Work out the finished part from the listing and answer in its coordinate system (mm). Face numbers are marked on the shaded views. A direction names the side the tool comes from. Give positions to 0.01 mm unless a question says otherwise; leave off trailing zeros. Loops run counter-clockwise (first coordinate to the right, second up) from the corner with the lowest first, then second, coordinate; pieces in that order, holes last. Notation, with made-up numbers: (54.5, 68.5) - (66.5, 68.5) arc R8 cw to (66.5, 80.5) - close; hole circle Ø4 at (60, 33). An arc over 180 degrees is marked (long way). One line per item, written item: value.
from build123d import *

# Parameters (mm, degrees)
F3_R          = 2.5
F4_DEPTH      = 42.28
F4_DEPTH_BACK = 29.68
F5_DEPTH      = 30
F5_DEPTH_BACK = 29.68
F3_W          = 18.04
F3_H          = 15.5
F3_R_2        = 5.32
F8_DEPTH      = 30
F9_START      = -20
F1_R          = 5.32
F1_R_2        = 3.41
F9_DEPTH      = 10
F10_R         = 4
F12_DEPTH     = 56.231
F14_DEPTH     = 74.271


# Not quite as in the source:
# - a feature of the source that left no trace in its solid (it failed there, or was rolled back) is left out


with BuildPart() as f4:
    # F3 (on Front) → F4 (new body, two sides)
    with BuildSketch(Plane.XZ) as f4_sk:
        with BuildLine():
            Line((-18.2932555878, -5.28), (-28.115, -5.28))
            Line((-28.115, -5.28), (-28.115, -28.115))
            Line((-28.115, -28.115), (28.115, -28.115))
            Line((28.115, -28.115), (28.115, -5.28))
            Line((28.115, -5.28), (18.2932555878, -5.28))
            ThreePointArc((18.2932555878, -5.28), (0, -19.04), (-18.2932555878, -5.28))
        make_face()
        with Locations((-23.62, -23.62)):
            Circle(F3_R, mode=Mode.SUBTRACT)
        with Locations((23.62, -23.62)):
            Circle(F3_R, mode=Mode.SUBTRACT)
    extrude(amount=-F4_DEPTH)
    extrude(f4_sk.sketch, amount=F4_DEPTH_BACK)

    # F3 (on Front) → F5 (join, two sides)
    with BuildSketch(Plane.XZ) as f5_sk:
        with BuildLine():
            Line((28.115, 28.115), (-28.115, 28.115))
            Line((-28.115, 28.115), (-28.115, 23.62))
            Line((-28.115, 23.62), (-28.115, 8.12))
            Line((-28.115, 8.12), (-28.115, -5.28))
            Line((-28.115, -5.28), (-18.2932555878, -5.28))
            ThreePointArc((-18.2932555878, -5.28), (-2.6662720799, 18.8523895885), (19.04, 0))
            ThreePointArc((19.04, 0), (18.8523895885, -2.6662720799), (18.2932555878, -5.28))
            Line((18.2932555878, -5.28), (28.115, -5.28))
            Line((28.115, -5.28), (28.115, 8.12))
            Line((28.115, 8.12), (28.115, 23.62))
            Line((28.115, 23.62), (28.115, 28.115))
        make_face()
        with Locations((-23.62, 23.62)):
            Circle(F3_R, mode=Mode.SUBTRACT)
        with Locations((23.62, 23.62)):
            Circle(F3_R, mode=Mode.SUBTRACT)
    extrude(amount=-F5_DEPTH)
    extrude(f5_sk.sketch, amount=F5_DEPTH_BACK)

    # F3 (on Front) → F8 (join)
    with BuildSketch(Plane.XZ):
        with Locations((37.135, 15.87)):
            Rectangle(F3_W, F3_H)
        with Locations((35.915, 15.87)):
            Circle(F3_R_2, mode=Mode.SUBTRACT)
        with Locations((-37.135, 15.87)):
            Rectangle(F3_W, F3_H)
        with Locations((-35.915, 15.87)):
            Circle(F3_R_2, mode=Mode.SUBTRACT)
    extrude(amount=-F8_DEPTH)

    # F1 (on Front) → F9 (join)
    with BuildSketch(Plane.XZ.offset(F9_START)):
        with Locations((35.915, 15.87)):
            Circle(F1_R)
        with Locations((35.915, 15.87)):
            Circle(F1_R_2, mode=Mode.SUBTRACT)
        with Locations((-35.915, 15.87)):
            Circle(F1_R)
        with Locations((-35.915, 15.87)):
            Circle(F1_R_2, mode=Mode.SUBTRACT)
    extrude(amount=-F9_DEPTH)

    # F10
    f10_edges = [f4.edges().sort_by_distance(p)[0] for p in [
        (-46.155, 15, 23.62),
        (-46.155, 15, 8.12),
        (-28.115, 6.3, -28.115),
        (28.115, 6.3, -28.115),
        (46.155, 15, 8.12),
        (46.155, 15, 23.62),
        (28.115, 0.16, 28.115),
        (-28.115, 0.16, 28.115),
    ]]
    fillet(f10_edges, radius=F10_R)

    # F11 (on face) → F12 (cut, through all)
    with BuildSketch(Plane.XY.offset(28.115)):
        with BuildLine():
            Line((16.115, 26), (-16.115, 26))
            ThreePointArc((-16.115, 26), (-18.9434271247, 24.8284271247), (-20.115, 22))
            Line((-20.115, 22), (-20.115, -21.68))
            ThreePointArc((-20.115, -21.68), (-18.9434271247, -24.5084271247), (-16.115, -25.68))
            Line((-16.115, -25.68), (16.115, -25.68))
            ThreePointArc((16.115, -25.68), (18.9434271247, -24.5084271247), (20.115, -21.68))
            Line((20.115, -21.68), (20.115, 22))
            ThreePointArc((20.115, 22), (18.9434271247, 24.8284271247), (16.115, 26))
        make_face()
    extrude(amount=-F12_DEPTH, mode=Mode.SUBTRACT)

    # F13 (on face) → F14 (cut, through all)
    with BuildSketch(Plane.YZ.offset(28.115)):
        with BuildLine():
            Line((22, 4.12), (-21.68, 4.12))
            ThreePointArc((-21.68, 4.12), (-24.5084271247, 2.9484271247), (-25.68, 0.12))
            Line((-25.68, 0.12), (-25.68, -16.115))
            ThreePointArc((-25.68, -16.115), (-24.5084271247, -18.9434271247), (-21.68, -20.115))
            Line((-21.68, -20.115), (22, -20.115))
            ThreePointArc((22, -20.115), (24.8284271247, -18.9434271247), (26, -16.115))
            Line((26, -16.115), (26, 0.12))
            ThreePointArc((26, 0.12), (24.8284271247, 2.9484271247), (22, 4.12))
        make_face()
    extrude(amount=-F14_DEPTH, mode=Mode.SUBTRACT)


solid = f4.part
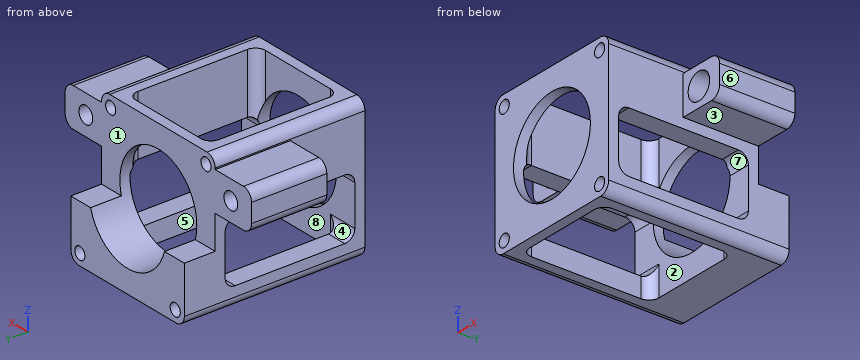
1. Section B-B (x = -23) is taken. Write down the section's boundary in (y, z) (3 decimals), and give its area (3 significant figures).
Output:
outline: (-29.68, -28.115) - (42.28, -28.115) - (42.28, -26.042) - (-29.68, -26.042) - close; (-29.68, -21.198) - (42.28, -21.198) - (42.28, -5.28) - (30, -5.28) - (30, 21.198) - (-29.68, 21.198) - close; (-29.68, 26.042) - (30, 26.042) - (30, 28.115) - (-29.68, 28.115) - close; hole (-25.68, -16.115) arc R4 ccw to (-21.68, -20.115) - (22, -20.115) arc R4 ccw to (26, -16.115) - (26, 0.12) arc R4 ccw to (22, 4.12) - (-21.68, 4.12) arc R4 ccw to (-25.68, 0.12) - close
area: 1,760 mm²
2. Section A-A (y = 34) is taken. Write down the section's boundary in (x, z) (3 decimals).
Output:
outline: (-28.115, -24.115) arc R4 ccw to (-24.115, -28.115) - (24.115, -28.115) arc R4 ccw to (28.115, -24.115) - (28.115, -5.28) - (18.293, -5.28) arc R19.04 cw to (-18.293, -5.28) - (-28.115, -5.28) - close; hole circle Ø5 at (-23.62, -23.62); hole circle Ø5 at (23.62, -23.62)
3. Flat-ended cylindrical pins translate along their axes: pin 1 Ø19 at (y, z) = (1, 11) entering from -X (3 decimals); pin 2 Ø11.5 at (x, z) = (-35.5, 14) entering from -Y; pin 3 Ø1.5 at (y, z) = (-13, 22) entering from +X (3 decimals); pin 4 Ø3 at (y, z) = (-19, 19.5) entering from -X (3 decimals). Find the tip coordinate at first contact, or state that the pin passes through.
Output:
pin 1: stops at x = -46.155
pin 2: stops at y = 0
pin 3: stops at x = 28.115
pin 4: stops at x = -28.115
4. The mould has two halves that part along X. Classify the marked faces 6, 7 and 8: released by +X, released by -X, zero draft, split by the parting line, or undercut.
Output:
face 6: released by +X
face 7: zero draft
face 8: undercut
5. Section D-D (y = -23) is taken. Write down the section's boundary in (x, z) (3 decimals), and give its area (3 significant figures).
Output:
outline: (-28.115, -24.115) arc R4 ccw to (-24.115, -28.115) - (-19.891, -28.115) - (-19.891, -19.891) - (-28.115, -19.891) - close; (-28.115, 3.896) - (-19.891, 3.896) - (-19.891, 28.115) - (-24.115, 28.115) arc R4 ccw to (-28.115, 24.115) - close; (19.891, -28.115) - (24.115, -28.115) arc R4 ccw to (28.115, -24.115) - (28.115, -19.891) - (19.891, -19.891) - close; (19.891, 3.896) - (28.115, 3.896) - (28.115, 24.115) arc R4 ccw to (24.115, 28.115) - (19.891, 28.115) - close; hole circle Ø5 at (-23.62, -23.62); hole circle Ø5 at (-23.62, 23.62); hole circle Ø5 at (23.62, -23.62); hole circle Ø5 at (23.62, 23.62)
area: 441 mm²
6. For the marked faces 1, 2, 3, 4 and 5, determine the directions among +Z, -Z, +X, -X, +Y, -Y from which every point of the face is accessible in a straight line to the end or side of a thin tool.
Output:
face 1: +Z, +X, -X, +Y
face 2: none
face 3: -Z, +X, +Y, -Y
face 4: +X, -X
face 5: +Z, -Z
7. Find the intervals of material crossed by line 1 along Y through (x, z) = (-14, 14); line 2 along X through (y, z) = (-3.5, 7.5) (3 decimals); line 3 along X through (y, z) = (10.5, 11) (3 decimals), in increasing order.
Output:
line 1: y = -29.68 to -25.68, 26 to 30
line 2: x = -28.115 to -20.115, 20.115 to 28.115
line 3: x = -45.995 to -38.056, -33.774 to -20.115, 20.115 to 33.774, 38.056 to 45.995
8. Section C-C (z = -7) is taken. Write down the section's boundary in (x, y) (3 decimals), and give its area (3 significant figures).
Output:
outline: (-28.115, -29.68) - (-17.707, -29.68) - (-17.707, -25.68) - (-28.115, -25.68) - close; (-28.115, 26) - (-17.707, 26) - (-17.707, 42.28) - (-28.115, 42.28) - close; (17.707, -29.68) - (28.115, -29.68) - (28.115, -25.68) - (17.707, -25.68) - close; (17.707, 26) - (28.115, 26) - (28.115, 42.28) - (17.707, 42.28) - close
area: 422 mm²
